For this review, take the finished solid that the model builds, in its own axes (mm). A direction names the side the tool comes from. Give positions to 0.01 mm unless a question says otherwise; leave off trailing zeros. Order: outer loops, then holes, each group sorted by start corner. A loop starts at its lowest first (then second) coordinate and runs counter-clockwise, first axis right, second up. Notation, with made-up numbers: (84.5, 30.5) - (130.5, 30.5) arc R20 ccw to (130.5, 36.5) - close; hole circle Ø6 at (30, 37.5). An arc over 180 degrees is marked (long way). One line per item, written item: value.
```python
from build123d import *

# Parameters (mm, degrees)
SKETCH001_W     = 30
SKETCH001_H     = 60
POCKET_DEPTH    = 15
SKETCH002_W     = 7.828685
SKETCH002_H     = 2.912844
POCKET001_DEPTH = 12.062428
SKETCH003_W     = 7.191467
SKETCH003_H     = 2.548873
POCKET002_DEPTH = 12.062428


with BuildPart() as part:
    # Sketch → Revolution (revolve)
    with BuildSketch(Plane.XY):
        with BuildLine():
            ThreePointArc((-26.469681, 17.367976), (-37.995377, 12.046633), (-42, 0))
            Line((-42, 0), (0, 0))
            Line((0, 18), (0, 0))
            Line((-26.469681, 17.367976), (0, 18))
        make_face()
    revolve(axis=Axis((0, 0, 0), (0, 1, 0)))

    # Sketch001 → Pocket (cut)
    with BuildSketch(Plane.XZ):
        Rectangle(SKETCH001_W, SKETCH001_H)
    extrude(amount=-POCKET_DEPTH, mode=Mode.SUBTRACT)

    # Sketch002 → Pocket001 (cut, through all)
    with BuildSketch(Plane(origin=(0, 0, 30), x_dir=(1, 0, 0), z_dir=(0, 0, -1))):
        with Locations((9.123454, -0.709289)):
            Rectangle(SKETCH002_W, SKETCH002_H)
    extrude(amount=-POCKET001_DEPTH, mode=Mode.SUBTRACT)

    # Sketch003 → Pocket002 (cut, through all)
    with BuildSketch(Plane.XY.offset(-30)):
        with Locations((9.168967, 0.61833)):
            Rectangle(SKETCH003_W, SKETCH003_H)
    extrude(amount=-POCKET002_DEPTH, mode=Mode.SUBTRACT)


solid = part.part
```
(1) Wall thickness on line 1 (X direction, y = 1, z = 0.5); line 2 (X direction, y = 8.75, z = -10); line 3 (Z direction, x = 8.5, y = 12.25): over which ranges is each line inside the solid? List them lowest first. Write a range as from..to.
Answers below:
line 1: x = -42.05..-15, 15..42.05
line 2: x = -39.01..-15, 15..39.01
line 3: z = -36.84..-30, 30..36.84
(2) Draft analysis for pull direction X (two halves, no side actions). For faces 6 (the face through (28, 0, 1)), 7 (the face through (5.209, 1, 36)), state which applies: pulls with the +X half, pulls with the -X half, needs draft (parallel to the pull), parting line crosses it, or undercut.
Answers below:
face 6: needs draft
face 7: undercut
(3) Take a section at A-A (y = 12). Write out the cut boundary in (x, z).
Answers below:
outline: circle Ø76.07 at (0, 0); hole (-15, -30) - (15, -30) - (15, 30) - (-15, 30) - close
(4) For P1, Ø3, axis at x = 20, y = 16, coming from the +Z side; P2, Ø6, axis at y = 4, z = -6, coming from the +X side; P3, Ø0.9, axis at y = 1.5, z = -34.5, coming from the +X side, all flat-tipped, find the tip position at first contact; note any pin that passes through.
Answers below:
P1: stops at z = 29.19
P2: stops at x = 41.89
P3: stops at x = 24.69
(5) Take a section at B-B (y = 3.5). Write out the cut boundary in (x, z), then the cut area to 3 significant figures.
Answers below:
outline: circle Ø83.85 at (0, 0); hole (-15, -30) - (15, -30) - (15, 30) - (-15, 30) - close
area: 3,720 mm^2
(6) Machinability: for faces 1 (the face through (-0.59, 17.97, -1.14)), 2 (the face through (9, 2.166, 36)), 3 (the face through (-23, 0, 1)), 4 (the face through (12.765, 1, -35)), 5 (the face through (0, 7, -30)), which of the approach directions +Z, -Z, +X, -X, +Y, -Y give a long, thin tool a straight path to every point of the face, cutting with its end or side? Answer none if there is none.
Answers below:
face 1: +Y
face 2: +Z, -Y
face 3: +Z, -Z, +X, -X, -Y
face 4: +Z, -Z, -Y
face 5: -Y
